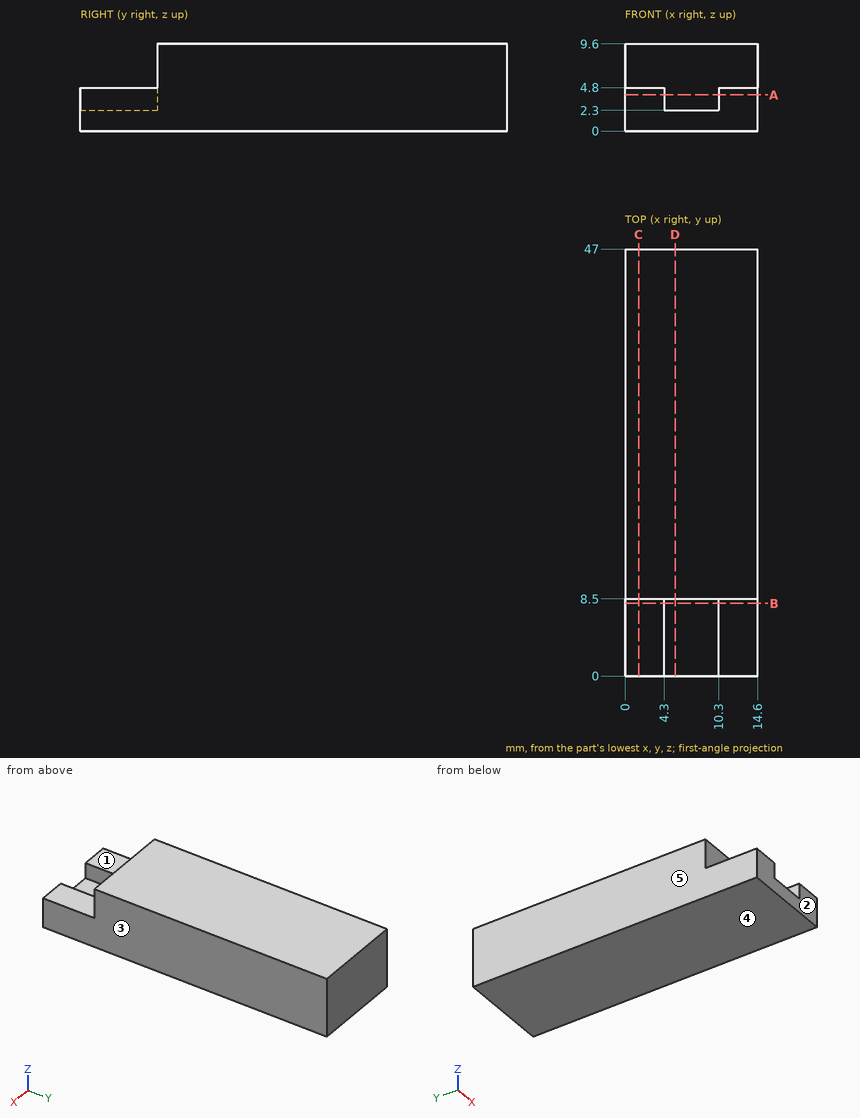
Verification items for this drawing (mm, ordinates from the low corner). A direction names the side the tool comes from. Coordinates: 2 decimals unless noted, no trailing zeros. Write each loop counter-clockwise with the first axis right and the second up, starting at its lowest first coordinate (ties: lowest second). Pieces come first, ordered by that corner, then holes. Notation, with made-up numbers: (-36, 79) -> (-8, 79) arc R19 ccw to (-8, 88) -> close; hole circle Ø3 at (68.25, 41.25). An arc over 180 degrees is marked (long way). Use CSV: the item, a comma, the result in double quotes. Start each with the question number.
Item 1: Cross-section at B-B, the plane y = 8. Record the cut outline in (x, z).
Item 2: Cross-section at A-A, the plane z = 4. Record the cut outline in (x, y), plus the area to 3 significant figures.
Item 3: Cross-section at D-D, the plane x = 5.5. Record the cut outline in (y, z), plus the area to 3 significant figures.
Item 4: Depth check by flat-ended pin: pin 1 Ø5 at (x, y) = (8.5, 2) entering from +Z. Enter the tip coordinate at first touch or a pass-through.
Item 5: Cross-section at C-C, the plane x = 1.5. Record the cut outline in (y, z).
Item 6: Thickness scan on line 1 (X direction, y = 8, z = 4); line 2 (Y direction, x = 2.25, z = 8.25); line 3 (Z direction, x = 7.5, y = 4.5). Record the ranges inside material, lowest first.
Item 7: Set-up check for the marked faces 1 and 2: record each of +Z, -Z, +X, -X, +Y, -Y from which the full face is reachable in a straight line by a thin tool's end or side.
Item 8: Mould release check, pull along X, two halves, no side actions. Record for the marked faces 3, 4 and 5: released by +X, released by -X, zero draft, split by the parting line, or undercut.
Answers:
1,outline,"(0, 0) -> (14.6, 0) -> (14.6, 4.8) -> (10.3, 4.8) -> (10.3, 2.3) -> (4.3, 2.3) -> (4.3, 4.8) -> (0, 4.8) -> close"
2,outline,"(0, 0) -> (4.3, 0) -> (4.3, 8.5) -> (10.3, 8.5) -> (10.3, 0) -> (14.6, 0) -> (14.6, 47) -> (0, 47) -> close"
2,area,"635 mm^2"
3,outline,"(0, 0) -> (47, 0) -> (47, 9.6) -> (8.5, 9.6) -> (8.5, 2.3) -> (0, 2.3) -> close"
3,area,"389 mm^2"
4,pin 1,"z = 4.8"
5,outline,"(0, 0) -> (47, 0) -> (47, 9.6) -> (8.5, 9.6) -> (8.5, 4.8) -> (0, 4.8) -> close"
6,line 1,"0 to 4.3, 10.3 to 14.6"
6,line 2,"8.5 to 47"
6,line 3,"0 to 2.3"
7,face 1,"+Z, +X, -X, -Y"
7,face 2,"+Z, -Z, +X, -X, -Y"
8,face 3,"released by +X"
8,face 4,"zero draft"
8,face 5,"released by -X"
